Autodesk Inventor part; units mm, degrees
ref_plane "YZ Plane" through (0, 0, 0) normal (1, 0, 0) x (0, 1, 0)
ref_plane "XZ Plane" through (0, 0, 0) normal (0, 1, 0) x (-1, 0, 0)
ref_plane "XY Plane" through (0, 0, 0) normal (0, 0, 1) x (1, 0, 0)
sketch "Sketch1" plane through (0, 0, 0) normal (0, 0, 1) x (1, 0, 0)
  line L0 (0, 0) -> (34, 0)
  line L1 (34, 0) -> (34, 16)
  line L2 (34, 16) -> (0, 16)
  line L3 (0, 16) -> (0, 0)
  line L4 (-4, 13) -> (0, 13)
  line L5 (0, 13) -> (0, 3)
  line L6 (0, 3) -> (-4, 3)
  line L7 (-4, 3) -> (-4, 13)
  line L8 (-4, 13) -> (0, 3) construction
  line L9 (0, 13) -> (-4, 3) construction
  line L10 (38, 13) -> (34, 13)
  line L11 (34, 13) -> (34, 3)
  line L12 (34, 3) -> (38, 3)
  line L13 (38, 3) -> (38, 13)
  line L14 (38, 13) -> (34, 3) construction
  line L15 (34, 13) -> (38, 3) construction
  point P0 (-2, 8)
  point P1 (36, 8)
  point P2 (0, 8)
  point P3 (0, 8)
  point P4 (0, 13)
  dimension "d0" = 34
  dimension "d1" = 16
  dimension "d2" = 4
  dimension "d3" = 4
  dimension "d4" = 10
  dimension "d5" = 10
extrude "Extrusion1" add sketch "Sketch1" along normal blind 3
properties part number "Frontrail"
Can you work these out from the model? Positions are in its coordinate system, mm. A direction names the side the tool comes from. Round coordinates to 2 decimals unless told otherwise and drop trailing zeros. Order: outer loops, then holes, each group sorted by start corner. A loop starts at its lowest first (then second) coordinate and runs counter-clockwise, first axis right, second up. Notation, with made-up numbers: M 62,37 L 69,37 A14 ccw 69,53 Z; hole C 48,17 d4. An arc over 180 degrees is marked long. Use a Markdown table: item, result.
1) Imagine slicing it at B-B (y = 13.5). List the corners of the cut face in (x, z) for me, then the cut area to 3 significant figures.
Geometry says:
| item | result |
|---|---|
| outline | M 0,0 L 34,0 L 34,3 L 0,3 Z |
| area | 102 mm² |
2) I'm going to push flat-ended pins straight in: P1, Ø0.9, axis at y = 14.5, z = 1.5, coming from the +X side; P2, Ø1.5, axis at x = -1.5, z = 2, coming from the +Y side; P3, Ø0.9, axis at x = 37, z = 1, coming from the -Y side. Where does each tip first touch, or does it pass through?
Geometry says:
| item | result |
|---|---|
| P1 | stops at x = 34 |
| P2 | stops at y = 13 |
| P3 | stops at y = 3 |
3) If I drill on line 1 along X through (y, z) = (2.5, 2.45); line 2 along Y through (x, z) = (34.5, 2), over which ranges is the centre line in solid material (lowest first)?
Geometry says:
| item | result |
|---|---|
| line 1 | x = 0 to 34 |
| line 2 | y = 3 to 13 |
4) On a 3-axis mill with a long thin cutter (end or side, diameter ignored), from which of +Z, -Z, +X, -X, +Y, -Y can I reach the whole of each face in a straight line? I mean faces 1 (the face through (36, 13, 1)), 2 (the face through (36, 3, 1)), 3 (the face through (-2, 3, 1)), 4 (the face through (17, 16, 1)), 5 (the face through (-2, 13, 1)). Say none if no direction works.
Geometry says:
| item | result |
|---|---|
| face 1 | +Z, -Z, +X, +Y |
| face 2 | +Z, -Z, +X, -Y |
| face 3 | +Z, -Z, -X, -Y |
| face 4 | +Z, -Z, +X, -X, +Y |
| face 5 | +Z, -Z, -X, +Y |
5) Imagine slicing it at A-A (z = 0.6). List the corners of the cut face in (x, y) for me.
Geometry says:
| item | result |
|---|---|
| outline | M -4,3 L 0,3 L 0,0 L 34,0 L 34,3 L 38,3 L 38,13 L 34,13 L 34,16 L 0,16 L 0,13 L -4,13 Z |
